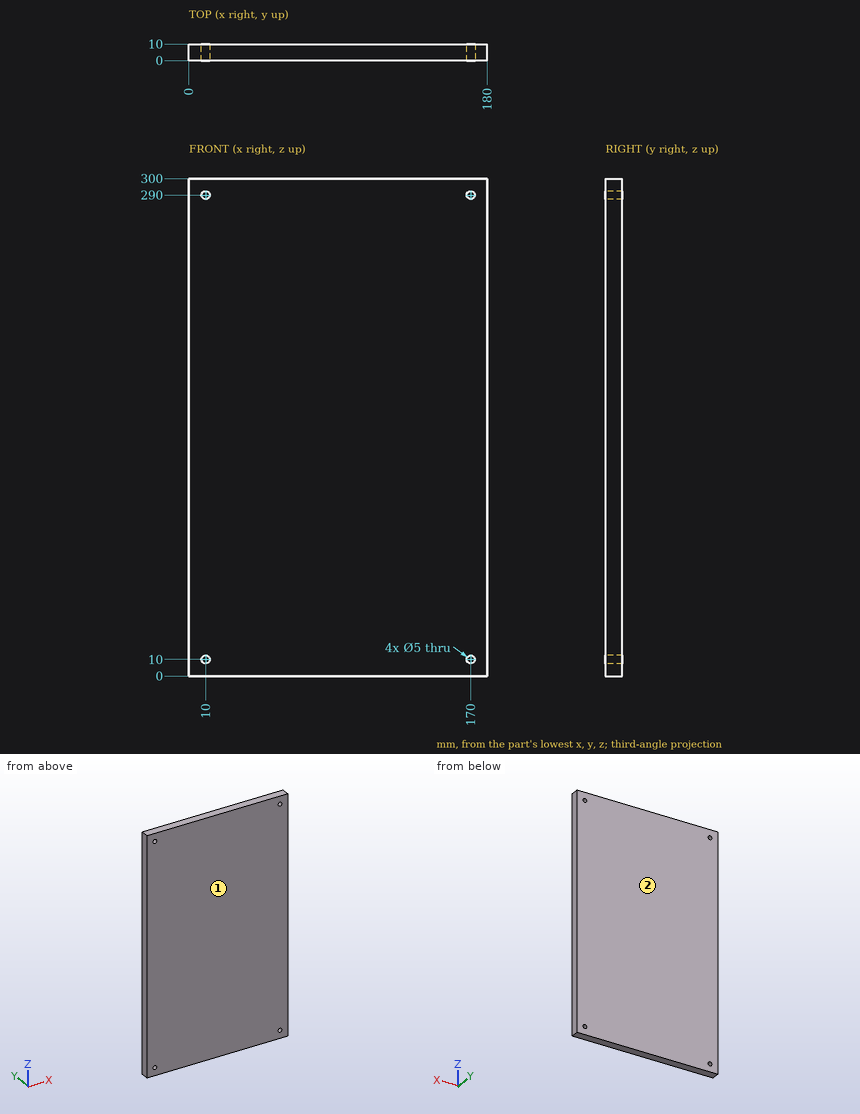
Verification items for this drawing (mm, ordinates from the low corner). Give positions to 0.01 mm unless a question says otherwise; leave off trailing zeros.
1) Gauge pin test, flat end, axial feed: pin 1 (3 mm diameter, centred on x = 10, z = 290, fed in from +Y). Record the tip position at first contact, or that the pin passes through.
2) Release check for a two-part mould opening along Y. For the marked faces 1 and 2 record: pulls with the +Y half, pulls with the -Y half, needs draft (parallel to the pull), parting line crosses it, or undercut.
3) Material ranges on L1, parallel to Z at x = 10, y = 3.25; L2, parallel to Z at x = 10.5, y = 7.75; L3, parallel to X at y = 6.25, z = 290, recorded low to high.
Computed:
1. pin 1: passes through
2. face 1: pulls with the -Y half
2. face 2: pulls with the +Y half
3. L1: z = 0 to 7.5, 12.5 to 287.5, 292.5 to 300
3. L2: z = 0 to 7.55, 12.45 to 287.55, 292.45 to 300
3. L3: x = 0 to 7.5, 12.5 to 167.5, 172.5 to 180
